Work out the finished part from the listing and answer in its coordinate system (mm). A direction names the side the tool comes from. Coordinates: 2 decimals unless noted, no trailing zeros. Write each loop counter-clockwise with the first axis right and the second up, starting at its lowest first coordinate (ties: lowest second). Pieces come first, ordered by that corner, then holes. Notation, with made-up numbers: (44.25, 55) - (55.25, 55) arc R22 cw to (55.25, 83) - close; hole circle Ø7 at (45, 85.5). An arc over 180 degrees is marked (long way). Use CSV: the item, a comma, the result in double quotes. Start each with the question number.
from build123d import *

# Parameters (mm, degrees)
ESQUISSE1_R             = 1.25
BOSS_EXTRU_1_DEPTH      = 12
ESQUISSE2_R             = 2.25
BOSS_EXTRU_2_DEPTH      = 1.9
ENL_V_MAT_EXTRU_1_DEPTH = 1


with BuildPart() as part:
    # Esquisse1 → Boss.-Extru.1 (new body)
    with BuildSketch(Plane.XY):
        Circle(ESQUISSE1_R)
    extrude(amount=BOSS_EXTRU_1_DEPTH)

    # Esquisse2 → Boss.-Extru.2 (add)
    with BuildSketch(Plane.XY.offset(12)):
        with Locations(Location((0, 0, 0), (0, 0, 180))):
            Circle(ESQUISSE2_R)
    extrude(amount=BOSS_EXTRU_2_DEPTH)

    # Esquisse3 → Enlèv. mat.-Extru.1 (cut)
    with BuildSketch(Plane.XY.offset(13.9)):
        Polygon((1.154700538, 0), (0.577350269, 1), (-0.577350269, 1), (-1.154700538, 0), (-0.577350269, -1), (0.577350269, -1), align=None)
    extrude(amount=-ENL_V_MAT_EXTRU_1_DEPTH, mode=Mode.SUBTRACT)


solid = part.part
Item 1: A cutting plane is placed at D-D (x = 1.95). Determine the outline of the cut face in (y, z), then the cut area to 3 significant figures.
Item 2: Determine the mould class of faces 1 (the face through (-1, -1, 13.9)), 2 (the face through (-0.87, -0.49, 13.41)), 3 (the face through (-0.27, -1.22, 5.92)) for opening direction Y: +Y half, -Y half, draft (parallel to the pull), parting line (faces both ways), or undercut.
Item 3: Each of these flat-tipped pins is pushed along its axis until it touches: pin 1 (1.5 mm diameter, centred on x = 0, z = 8, fed in from +Y); pin 2 (0.6 mm diameter, centred on x = 0, y = 0, fed in from +Z). Where does it stop, or does it pass through?
Item 4: Straight lines are drawn through the part: probe 1 along Z at (x, y) = (-1, 1.35); probe 2 along Y at (x, z) = (0.05, 2); probe 3 along Z at (x, y) = (-0.5, 0.65). For each, find the intervals that lie inside material, in ascending order. Write a range as [from, to].
Item 5: A cutting plane is placed at A-A (x = 0). Determine the outline of the cut face in (y, z), then the cut area to 4 significant figures.
Item 6: A cutting plane is placed at B-B (y = 0.15). Determine the outline of the cut face in (x, z) (3 decimals).
Item 7: Which of the six approach directions +Z, -Z, +X, -X, +Y, -Y give full straight-line access (tool end or side, diameter ignored) to faces 4 (the face through (0.87, 0.49, 13.41)), 5 (the face through (-1, 1, 12)), 6 (the face through (1.66, -1.52, 12.94))?
Item 8: A cutting plane is placed at C-C (z = 6.5). Determine the outline of the cut face in (x, y).
Calculated:
1,outline,"(-1.12, 12) - (1.12, 12) - (1.12, 13.9) - (-1.12, 13.9) - close"
1,area,"4.27 mm²"
2,face 1,"draft"
2,face 2,"undercut"
2,face 3,"parting line"
3,pin 1,"stops at y = 1.25"
3,pin 2,"stops at z = 12.9"
4,probe 1,"z = [12, 13.9]"
4,probe 2,"y = [-1.25, 1.25]"
4,probe 3,"z = [0, 12.9]"
5,outline,"(-2.25, 12) - (-1.25, 12) - (-1.25, 0) - (1.25, 0) - (1.25, 12) - (2.25, 12) - (2.25, 13.9) - (1, 13.9) - (1, 12.9) - (-1, 12.9) - (-1, 13.9) - (-2.25, 13.9) - close"
5,area,"36.55 mm²"
6,outline,"(-2.245, 12) - (-1.241, 12) - (-1.241, 0) - (1.241, 0) - (1.241, 12) - (2.245, 12) - (2.245, 13.9) - (1.068, 13.9) - (1.068, 12.9) - (-1.068, 12.9) - (-1.068, 13.9) - (-2.245, 13.9) - close"
7,face 4,"+Z"
7,face 5,"-Z"
7,face 6,"+Z, -Z"
8,outline,"circle Ø2.5 at (0, 0)"
